Geometry: final body of the model. Coordinates: model frame, mm. A direction names the side the tool comes from. Coordinates: 2 decimals unless noted, no trailing zeros. Order: outer loops, then holes, each group sorted by start corner. A loop starts at its lowest first (then second) coordinate and runs counter-clockwise, first axis right, second up. Notation, with made-up numbers: (19, 69) -> (50, 69) arc R23 cw to (50, 88) -> close; hole circle Ø7 at (57.5, -24). An arc over 180 degrees is marked (long way). Use one line per item in the form item = value.
```python
from build123d import *

# Parameters (mm, degrees)
SKETCH1_W              = 278.049859422
SKETCH1_H              = 166.000659628
BOSS_EXTRUDE1_DEPTH    = 24
SKETCH2_W              = 189.719631187
SKETCH2_H              = 145.09871859
CUT_EXTRUDE1_DEPTH     = 325.721331793
SKETCH3_W              = 272.049859422
SKETCH3_H              = 160.000659628
CUT_EXTRUDE2_DEPTH     = 20
FILLET1_R              = 50
FILLET2_R              = 50
SKETCH4_W              = 68.204970116
SKETCH4_H              = 3
BOSS_EXTRUDE2_DEPTH    = 20
FILLET4_R              = 20
FILLET5_R              = 20
SKETCH5_W              = 66.657615254
SKETCH5_H              = 3
BOSS_EXTRUDE3_DEPTH    = 20
FILLET6_R              = 20
FILLET7_R              = 20
SKETCH6_R              = 2.75
HOLESFORBOLTS1_DEPTH   = 326.295157302
SKETCH7_R              = 2.75
CUT_EXTRUDE4_DEPTH     = 327.808725896
SKETCH8_R              = 2.75
CUT_EXTRUDE5_DEPTH     = 20
SKETCH11_W             = 13.646136269
SKETCH11_H             = 11.541733762
CUT_EXTRUDE6_DEPTH     = 327.808725896
SKETCH12_W             = 8.844116654
SKETCH12_H             = 9.360207276
CUT_EXTRUDE7_DEPTH     = 327.808725896
HOLESINLIDFORPICOVER_R = 2.75
CUT_EXTRUDE8_DEPTH     = 107.252842694
LIDHOLESFORPI_R        = 1.455
CUT_EXTRUDE9_DEPTH     = 4
SKETCH14_R             = 2.75
CUT_EXTRUDE10_DEPTH    = 4


with BuildPart() as part:
    # Sketch1 → Boss-Extrude1 (new body)
    with BuildSketch(Plane(origin=(0, 0, 0), x_dir=(1, 0, 0), z_dir=(0, 1, 0))):
        with Locations((139.024929711, 83.000329814)):
            Rectangle(SKETCH1_W, SKETCH1_H)
    extrude(amount=BOSS_EXTRUDE1_DEPTH)

    # Sketch2 → Cut-Extrude1 (cut, through all)
    with BuildSketch(Plane(origin=(0, 0, 0), x_dir=(-1, 0, 0), z_dir=(0, -1, 0))):
        with Locations((-80.61962524, 84.091093057)):
            Rectangle(SKETCH2_W, SKETCH2_H)
    extrude(amount=-CUT_EXTRUDE1_DEPTH, mode=Mode.SUBTRACT)

    # Sketch3 → Cut-Extrude2 (cut)
    with BuildSketch(Plane(origin=(0, 24, 0), x_dir=(1, 0, 0), z_dir=(0, 1, 0))):
        with Locations((139.024929711, 83.000329814)):
            Rectangle(SKETCH3_W, SKETCH3_H)
    extrude(amount=-CUT_EXTRUDE2_DEPTH, mode=Mode.SUBTRACT)

    # Fillet1
    fillet1_edges = [part.edges().sort_by_distance(p)[0] for p in [
        (175.479440834, 2, -11.541733762),
    ]]
    fillet(fillet1_edges, radius=FILLET1_R)

    # Fillet2
    fillet2_edges = [part.edges().sort_by_distance(p)[0] for p in [
        (175.479440834, 2, -156.640452352),
    ]]
    fillet(fillet2_edges, radius=FILLET2_R)

    # Sketch4 → Boss-Extrude2 (add)
    with BuildSketch(Plane(origin=(0, 24, 0), x_dir=(1, 0, 0), z_dir=(0, 1, 0))):
        with Locations((137.24279725, 1.5)):
            Rectangle(SKETCH4_W, SKETCH4_H)
    extrude(amount=BOSS_EXTRUDE2_DEPTH)

    # Fillet4
    fillet4_edges = [part.edges().sort_by_distance(p)[0] for p in [
        (103.140312192, 24, -1.5),
    ]]
    fillet(fillet4_edges, radius=FILLET4_R - 0.0001)  # a hair under: the kernel refuses the full size

    # Fillet5
    fillet5_edges = [part.edges().sort_by_distance(p)[0] for p in [
        (171.345282308, 24, -1.5),
    ]]
    fillet(fillet5_edges, radius=FILLET5_R - 0.0001)  # a hair under: the kernel refuses the full size

    # Sketch5 → Boss-Extrude3 (add)
    with BuildSketch(Plane(origin=(0, 24, 0), x_dir=(1, 0, 0), z_dir=(0, 1, 0))):
        with Locations((137.51551703, 164.500659628)):
            Rectangle(SKETCH5_W, SKETCH5_H)
    extrude(amount=BOSS_EXTRUDE3_DEPTH)

    # Fillet6
    fillet6_edges = [part.edges().sort_by_distance(p)[0] for p in [
        (104.186709403, 24, -164.500659628),
    ]]
    fillet(fillet6_edges, radius=FILLET6_R - 0.0001)  # a hair under: the kernel refuses the full size

    # Fillet7
    fillet7_edges = [part.edges().sort_by_distance(p)[0] for p in [
        (170.844324657, 24, -164.500659628),
    ]]
    fillet(fillet7_edges, radius=FILLET7_R - 0.0001)  # a hair under: the kernel refuses the full size

    # Sketch6 → HolesForBolts1 (cut, through all)
    with BuildSketch(Plane.XY.offset(-163.000659628)):
        with Locations((151.506445743, 20.306027196)):
            Circle(SKETCH6_R)
        with Locations((117.392557181, 20.306027196)):
            Circle(SKETCH6_R)
    extrude(amount=-HOLESFORBOLTS1_DEPTH, mode=Mode.SUBTRACT)

    # Sketch7 → Cut-Extrude4 (cut, through all)
    with BuildSketch(Plane(origin=(0, 0, -166.000659628), x_dir=(-1, 0, 0), z_dir=(0, 0, -1))):
        with Locations((-23.654153003, 11.675842417)):
            Circle(SKETCH7_R)
        with Locations((-55.441477074, 11.675842417)):
            Circle(SKETCH7_R)
        with Locations((-83.004388954, 11.675842417)):
            Circle(SKETCH7_R)
        with Locations((-184.727610529, 11.675842417)):
            Circle(SKETCH7_R)
        with Locations((-222.645451091, 11.675842417)):
            Circle(SKETCH7_R)
        with Locations((-255.881733076, 11.675842417)):
            Circle(SKETCH7_R)
    extrude(amount=-CUT_EXTRUDE4_DEPTH, mode=Mode.SUBTRACT)

    # Sketch8 → Cut-Extrude5 (cut)
    with BuildSketch(Plane(origin=(0, 0, -3), x_dir=(-1, 0, 0), z_dir=(0, 0, -1))):
        with Locations((-120.487078085, 23.280365191)):
            Circle(SKETCH8_R)
        with Locations((-152.966291723, 23.280365191)):
            Circle(SKETCH8_R)
    extrude(amount=-CUT_EXTRUDE5_DEPTH, mode=Mode.SUBTRACT)

    # Sketch11 → Cut-Extrude6 (cut, through all)
    with BuildSketch(Plane.XZ):
        with Locations((6.823068135, -5.770866881)):
            Rectangle(SKETCH11_W, SKETCH11_H)
    extrude(amount=-CUT_EXTRUDE6_DEPTH, mode=Mode.SUBTRACT)

    # Sketch12 → Cut-Extrude7 (cut, through all)
    with BuildSketch(Plane.XZ):
        with Locations((4.422058327, -161.32055599)):
            Rectangle(SKETCH12_W, SKETCH12_H)
    extrude(amount=-CUT_EXTRUDE7_DEPTH, mode=Mode.SUBTRACT)

    # HolesInLidForPiCover → Cut-Extrude8 (cut)
    with BuildSketch(Plane.XZ):
        with Locations(Location((223.013799051, -141.608636884, 0), (0, 0, 270))):
            Circle(HOLESINLIDFORPICOVER_R)
        with Locations(Location((223.013799051, -22.129735073, 0), (0, 0, 270))):
            Circle(HOLESINLIDFORPICOVER_R)
    extrude(amount=-CUT_EXTRUDE8_DEPTH, mode=Mode.SUBTRACT)

    # LidHolesForPi → Cut-Extrude9 (cut)
    with BuildSketch(Plane.XZ):
        with Locations(Location((200.562123112, -102.370703816, 0), (0, 0, 270))):
            Circle(LIDHOLESFORPI_R)
        with Locations(Location((200.562123112, -53.502923562, 0), (0, 0, 270))):
            Circle(LIDHOLESFORPI_R)
        with Locations(Location((258.544947711, -53.502923562, 0), (0, 0, 270))):
            Circle(LIDHOLESFORPI_R)
        with Locations(Location((258.544947711, -102.370703816, 0), (0, 0, 270))):
            Circle(LIDHOLESFORPI_R)
    extrude(amount=-CUT_EXTRUDE9_DEPTH, mode=Mode.SUBTRACT)

    # Sketch14 → Cut-Extrude10 (cut)
    with BuildSketch(Plane.XZ):
        with Locations(Location((264.763568483, -18.920123653, 0), (0, 0, 270))):
            Circle(SKETCH14_R)
        with Locations(Location((181.616848195, -18.918729826, 0), (0, 0, 270))):
            Circle(SKETCH14_R)
    extrude(amount=-CUT_EXTRUDE10_DEPTH, mode=Mode.SUBTRACT)


solid = part.part
```
1) Pull-direction query (Z, two-part tool) for faces 1 (the flat face through (278.05, 12, -82)), 2 (the flat face through (142, 17, -166.001)), 3 (the cylindrical face through (160.444, 2.028, -25.8)); classes: released by +Z, released by -Z, zero draft, split by the parting line, or undercut.
Results found:
face_1 = zero draft
face_2 = released by -Z
face_3 = undercut
2) Material intervals for probe 1 along Z at (x, y) = (194.5, 10.5); probe 2 along X at (y, z) = (14, -126); probe 3 along Y at (x, z) = (235, -88), sorted ascending. Write a range as from..to.
Results found:
probe_1 = -166..-163, -3..0
probe_2 = 275.05..278.05
probe_3 = 0..4
3) Section B-B, the plane z = -141.5. Output: boundary loops of the cut face in (x, y).
Results found:
outline = (161.32, 0) -> (220.27, 0) -> (220.27, 4) -> (161.32, 4) -> close; (225.76, 0) -> (278.05, 0) -> (278.05, 24) -> (275.05, 24) -> (275.05, 4) -> (225.76, 4) -> close
4) Section A-A, the plane x = 110.5. Output: boundary loops of the cut face in (y, z), and give its area (3 significant figures).
Results found:
outline = (0, -166) -> (44, -166) -> (44, -163) -> (4, -163) -> (4, -156.64) -> (0, -156.64) -> close; (0, -11.54) -> (4, -11.54) -> (4, -3) -> (44, -3) -> (44, 0) -> (0, 0) -> close
area = 324 mm2
5) Section C-C, the plane y = 32. Output: boundary loops of the cut face in (x, z).
Results found:
outline = (99.14, -3) -> (175.35, -3) -> (175.35, 0) -> (99.14, 0) -> close; (100.19, -166) -> (174.84, -166) -> (174.84, -163) -> (100.19, -163) -> close
6) Section D-D, the plane x = 206.5. Output: boundary loops of the cut face in (y, z), and give its area (3 significant figures).
Results found:
outline = (0, -166) -> (24, -166) -> (24, -163) -> (4, -163) -> (4, -3) -> (24, -3) -> (24, 0) -> (0, 0) -> close
area = 784 mm2
7) Access query for faces 4 (the flat face through (140, 20, -163.001)), 5 (the cylindrical face through (120.016, 21.132, -164.48)), 6 (the cylindrical face through (161.221, 2.028, -141.605)), 7 (the cylindrical face through (155.714, 23.401, -1.521)). Directions: +Z, -Z, +X, -X, +Y, -Y. A direction counts if a zero-diameter tool reaches every point of the face in a straight line with its end or side. Return the directions, or none.
Results found:
face_4 = -X, +Y
face_5 = -Z
face_6 = -X, +Y, -Y
face_7 = +Z
8) Contact query for flat-ended pins moving along their axis: P1, Ø1.2, axis at y = 1.5, z = -87.5, coming from the -X side; P2, Ø10, axis at y = 15, z = -55.5, coming from the -X side. Output: stop coordinate, or through.
Results found:
P1 = 175.48
P2 = 275.05
